```python
from build123d import *

# Parameters (mm, degrees)
SKETCH_2_W          = 210
SKETCH_2_H          = 105
EXTRUDE_1_DEPTH     = 90
SKETCH_5_W          = 99
SKETCH_5_H          = 80
CUT_EXTRUDE_2_DEPTH = 200
SKETCH_6_W          = 75
SKETCH_6_H          = 45
EXTRUDE_2_DEPTH     = 50
SKETCH_7_W          = 69
SKETCH_7_H          = 40
CUT_EXTRUDE_3_DEPTH = 281.100428418
SKETCH_8_R          = 12
CUT_EXTRUDE_4_DEPTH = 170.724040725
SKETCH_9_R          = 2
CUT_EXTRUDE_5_DEPTH = 208.725780778
SKETCH_11_W         = 25
SKETCH_11_H         = 105
CUT_EXTRUDE_6_DEPTH = 30
SKETCH_4_R          = 11.5
CUT_EXTRUDE_8_DEPTH = 3


with BuildPart() as part:
    # 草图2 → 凸台-拉伸1 (new body)
    with BuildSketch(Plane(origin=(0, 0, 0), x_dir=(1, 0, 0), z_dir=(0, 1, 0))):
        Rectangle(SKETCH_2_W, SKETCH_2_H)
    extrude(amount=EXTRUDE_1_DEPTH)

    # 草图5 → 切除-拉伸2 (cut)
    with BuildSketch(Plane(origin=(105, 0, 0), x_dir=(0, 0, -1), z_dir=(1, 0, 0))):
        with Locations((0, 40)):
            Rectangle(SKETCH_5_W, SKETCH_5_H)
    extrude(amount=-CUT_EXTRUDE_2_DEPTH, mode=Mode.SUBTRACT)

    # 草图6 → 凸台-拉伸2 (add)
    with BuildSketch(Plane.ZY.offset(105)):
        with Locations((15, 22.5)):
            Rectangle(SKETCH_6_W, SKETCH_6_H)
    extrude(amount=EXTRUDE_2_DEPTH)

    # 草图7 → 切除-拉伸3 (cut, through all)
    with BuildSketch(Plane.ZY.offset(155)):
        with Locations((15, 20)):
            Rectangle(SKETCH_7_W, SKETCH_7_H)
    extrude(amount=-CUT_EXTRUDE_3_DEPTH, mode=Mode.SUBTRACT)

    # 草图8 → 切除-拉伸4 (cut, through all)
    with BuildSketch(Plane(origin=(0, 45, 0), x_dir=(1, 0, 0), z_dir=(0, 1, 0))):
        with Locations(Location((-130, -25.5, 0), (0, 0, 270))):
            Circle(SKETCH_8_R)
    extrude(amount=-CUT_EXTRUDE_4_DEPTH, mode=Mode.SUBTRACT)

    # 草图9 → 切除-拉伸5 (cut, through all)
    with BuildSketch(Plane.XY.offset(52.5)):
        with Locations((-70, 50)):
            Circle(SKETCH_9_R)
        with Locations((70, 50)):
            Circle(SKETCH_9_R)
    extrude(amount=-CUT_EXTRUDE_5_DEPTH, mode=Mode.SUBTRACT)

    # 草图11 → 切除-拉伸6 (cut)
    with BuildSketch(Plane(origin=(0, 90, 0), x_dir=(1, 0, 0), z_dir=(0, 1, 0))):
        with Locations((92.5, 0)):
            Rectangle(SKETCH_11_W, SKETCH_11_H)
    extrude(amount=-CUT_EXTRUDE_6_DEPTH, mode=Mode.SUBTRACT)

    # 草图4 → 切除-拉伸8 (cut)
    with BuildSketch(Plane(origin=(0, 90, 0), x_dir=(1, 0, 0), z_dir=(0, 1, 0))):
        with Locations(Location((-80.5, 33, 0), (0, 0, 270))):
            Circle(SKETCH_4_R)
        with Locations(Location((55.5, 33, 0), (0, 0, 270))):
            Circle(SKETCH_4_R)
        with Locations(Location((-80.5, -33, 0), (0, 0, 270))):
            Circle(SKETCH_4_R)
        with Locations(Location((55.5, -33, 0), (0, 0, 270))):
            Circle(SKETCH_4_R)
    extrude(amount=-CUT_EXTRUDE_8_DEPTH, mode=Mode.SUBTRACT)


solid = part.part
```
Design review of the part built by this model. Coordinates are the model's own, in mm. A direction names the side the tool comes from. Coordinates: 2 decimals unless noted, no trailing zeros. Order: outer loops, then holes, each group sorted by start corner. A loop starts at its lowest first (then second) coordinate and runs counter-clockwise, first axis right, second up.
1) Wall thickness on line 1 along X through (y, z) = (89.25, 33); line 2 along Z through (x, y) = (83, 12.5); line 3 along Y through (x, z) = (-21, -39): over which ranges is each line inside the solid? List them lowest first.
2) Take a section at D-D, the plane y = 68.5. Give the boundary of the cut face in (x, z).
3) Take a section at C-C, the plane z = -33. Give the boundary of the cut face in (x, y).
4) Take a section at A-A, the plane x = -110.5. Give the boundary of the cut face in (y, z), and give its area (3 significant figures).
5) Clearance check with flat-ended pins moving along their axes: pin 1 (3.5 mm diameter, centred on x = 93, z = -50.5, fed in from +Y); pin 2 (12 mm diameter, centred on y = 80.5, z = 15.5, fed in from -X); pin 3 (15 mm diameter, centred on x = -125, z = 1, fed in from +Y). State where each tip first meets the part, or that it passes through.
6) Mouldability with a two-part tool opening along X and no side actions: class faces 4 (the flat face through (80, 83, 0)), 5 (the flat face through (56, 87, -33)), 6 (the flat face through (-27, 39, 49.5)) as +X half, -X half, draft (parallel to the pull), parting line (faces both ways), or undercut.
7) For faces 1 (the flat face through (6, 39, -49.5)), 2 (the flat face through (-135, 45, 14)), 3 (the flat face through (-119, 40, 15)), list the 3-axis set-ups (+Z, -Z, +X, -X, +Y, -Y) from which the entire face can be reached by the end or side of a thin tool; tool diameter is ignored.
8) Take a section at B-B, the plane y = 18.5. Give the boundary of the cut face in (x, z).
Returned:
1. line 1: x = -105 to -92, -69 to 44, 67 to 80
1. line 2: z = -52.5 to -49.5, 49.5 to 52.5
1. line 3: y = 80 to 90
2. outline: (-105, -52.5) - (80, -52.5) - (80, -49.5) - (-95, -49.5) - (-95, 49.5) - (80, 49.5) - (80, 52.5) - (-105, 52.5) - close
3. outline: (-105, 0) - (-95, 0) - (-95, 80) - (80, 80) - (80, 90) - (67, 90) - (67, 87) - (44, 87) - (44, 90) - (-69, 90) - (-69, 87) - (-92, 87) - (-92, 90) - (-105, 90) - close
4. outline: (0, -22.5) - (45, -22.5) - (45, 52.5) - (0, 52.5) - (0, 49.5) - (40, 49.5) - (40, -19.5) - (0, -19.5) - close
4. area: 615 mm2
5. pin 1: stops at y = 60
5. pin 2: stops at x = -105
5. pin 3: stops at y = 45
6. face 4: +X half
6. face 5: undercut
6. face 6: draft
7. face 1: +X, -Y
7. face 2: +Z, -Z, -X, +Y
7. face 3: +X, -X, -Y
8. outline: (-155, -22.5) - (-105, -22.5) - (-105, -52.5) - (105, -52.5) - (105, -49.5) - (-95, -49.5) - (-95, -19.5) - (-155, -19.5) - close; (-155, 49.5) - (105, 49.5) - (105, 52.5) - (-155, 52.5) - close
